```python
from build123d import *

# Parameters (mm, degrees)
F0_W     = 48
F0_H     = 12
F1_DEPTH = 1
F3_R     = 1.5
F4_R     = 0.5
F6_DEPTH = 1
F5_R     = 1
F7_DEPTH = 0.5


with BuildPart() as f1:
    # F0 (on Top) → F1 (new body)
    with BuildSketch(Plane.XY):
        Rectangle(F0_W, F0_H)
    extrude(amount=F1_DEPTH)

    # F3
    f3_edges = [f1.edges().sort_by_distance(p)[0] for p in [
        (24, -6, 0.5),
        (24, 6, 0.5),
        (-24, 6, 0.5),
        (-24, -6, 0.5),
    ]]
    fillet(f3_edges, radius=F3_R)

    # F4 (on face) → F6 (cut)
    with BuildSketch(Plane.XY.offset(1)):
        with Locations((4, 4)):
            Circle(F4_R)
        with Locations((8, 4)):
            Circle(F4_R)
        with Locations((12, 4)):
            Circle(F4_R)
        with Locations((16, 4)):
            Circle(F4_R)
        with Locations((20, 4)):
            Circle(F4_R)
        with Locations((20, -4)):
            Circle(F4_R)
        with Locations((16, -4)):
            Circle(F4_R)
        with Locations((12, -4)):
            Circle(F4_R)
        with Locations((8, -4)):
            Circle(F4_R)
        with Locations((4, -4)):
            Circle(F4_R)
    extrude(amount=-F6_DEPTH, mode=Mode.SUBTRACT)

    # F5 (on face) → F7 (cut)
    with BuildSketch(Plane.XY.offset(1)):
        with Locations((4, 4)):
            Circle(F5_R)
        with Locations((8, 4)):
            Circle(F5_R)
        with Locations((12, 4)):
            Circle(F5_R)
        with Locations((16, 4)):
            Circle(F5_R)
        with Locations((20, 4)):
            Circle(F5_R)
        with Locations((20, -4)):
            Circle(F5_R)
        with Locations((16, -4)):
            Circle(F5_R)
        with Locations((12, -4)):
            Circle(F5_R)
        with Locations((8, -4)):
            Circle(F5_R)
        with Locations((4, -4)):
            Circle(F5_R)
    extrude(amount=-F7_DEPTH, mode=Mode.SUBTRACT)


solid = f1.part
```
The listing builds one solid part. Answer for the finished solid, in the listing's coordinates (mm). A direction names the side the tool comes from. Give positions to 0.01 mm unless a question says otherwise; leave off trailing zeros. Loops run counter-clockwise (first coordinate to the right, second up) from the corner with the lowest first, then second, coordinate; pieces in that order, holes last. Notation, with made-up numbers: (24.5, -16.75) - (82.5, -16.75) arc R36 ccw to (82.5, 22.25) - close; hole circle Ø7 at (51, 84). An arc over 180 degrees is marked (long way). Return JSON: item names as keys, results as strings. Group by question number.
1. Find section A-A (z = 0.25). State how many separate pieces and enclosed holes the cut face has, then the cut area to 3 significant figures.
2. Which of the six approach directions +Z, -Z, +X, -X, +Y, -Y give full straight-line access (tool end or side, diameter ignored) to faces 4 (the cylindrical face through (8.477, 4.15, 0.254)), 5 (the cylindrical face through (19.263, 4.676, 0.754))?
3. Find section B-B (x = 8). Write down the section's boundary in (y, z), then the cut area to 3 significant figures.
4. Given pin 1 Ø1.6 at (x, y) = (16, 4) entering from +Z, flat-ended and moving along its own axis, determine where the tip first touches the part or whether it passes through.
5. Determine the mould class of faces 1 (the cylindrical face through (7.263, 4.676, 0.754)), 2 (the flat face through (-24, -0.1, 0.5)), 3 (the cylindrical face through (23.55, -5.57, 0.51)) for opening direction X: pulls with the +X half, pulls with the -X half, needs draft (parallel to the pull), parting line crosses it, or undercut.
6. Straight lines are drawn through the part: line 1 (Y direction, x = 16, z = 0.8); line 2 (Y direction, x = 16, z = 0.15); line 3 (X direction, y = 4.25, z = 0.35). For each, find the intervals that lie inside material, in ascending order. Write a range as [from, to].
Verdict:
{
 "1": {"separate pieces": "1", "enclosed holes": "10", "area": "566 mm^2"},
 "2": {"face 4": "+Z, -Z", "face 5": "+Z"},
 "3": {"outline": "(-6, 0) - (-4.5, 0) - (-4.5, 0.5) - (-5, 0.5) - (-5, 1) - (-6, 1) - close; (-3.5, 0) - (3.5, 0) - (3.5, 0.5) - (3, 0.5) - (3, 1) - (-3, 1) - (-3, 0.5) - (-3.5, 0.5) - close; (4.5, 0) - (6, 0) - (6, 1) - (5, 1) - (5, 0.5) - (4.5, 0.5) - close", "area": "9.00 mm^2"},
 "4": {"pin 1": "stops at z = 0.5"},
 "5": {"face 1": "undercut", "face 2": "pulls with the -X half", "face 3": "pulls with the +X half"},
 "6": {"line 1": "y = [-6, -5], [-3, 3], [5, 6]", "line 2": "y = [-6, -4.5], [-3.5, 3.5], [4.5, 6]", "line 3": "x = [-24, 3.57], [4.43, 7.57], [8.43, 11.57], [12.43, 15.57], [16.43, 19.57], [20.43, 24]"}
}
